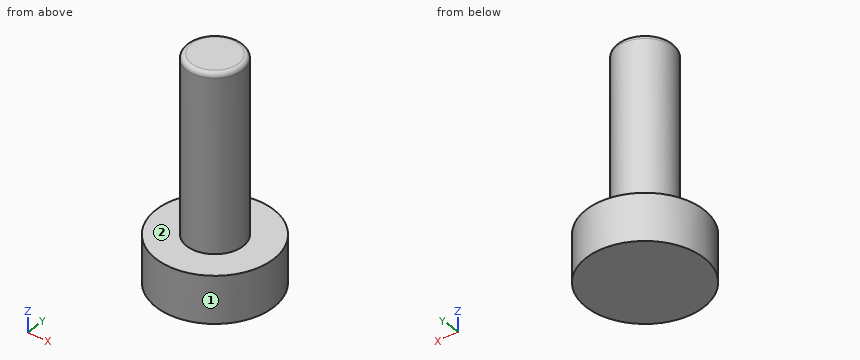
from build123d import *

# Parameters (mm, degrees)
ESQUISSE1_R        = 5
BOSS_EXTRU_1_DEPTH = 4
ESQUISSE2_R        = 2.4
BOSS_EXTRU_2_DEPTH = 15
CONG_1_R           = 0.4


with BuildPart() as part:
    # Esquisse1 → Boss.-Extru.1 (new body)
    with BuildSketch(Plane.XY):
        Circle(ESQUISSE1_R)
    extrude(amount=BOSS_EXTRU_1_DEPTH)

    # Esquisse2 → Boss.-Extru.2 (add)
    with BuildSketch(Plane.XY.offset(4)):
        Circle(ESQUISSE2_R)
    extrude(amount=BOSS_EXTRU_2_DEPTH)

    # Congé1
    cong_1_edges = [part.edges().sort_by_distance(p)[0] for p in [
        (-2.4, 0, 19),
    ]]
    fillet(cong_1_edges, radius=CONG_1_R)


solid = part.part
CAD build for the part. Positions are in the model's coordinates, mm. Face numbers are marked on the shaded views. A direction names the side the tool comes from. Round coordinates to 2 decimals unless told otherwise and drop trailing zeros. Write each loop counter-clockwise with the first axis right and the second up, starting at its lowest first coordinate (ties: lowest second). Pieces come first, ordered by that corner, then holes. Notation, with made-up numbers: M 68.25,14 L 116.25,14 A15 cw 116.25,31 Z; hole C 36.25,-19 d3. An arc over 180 degrees is marked long. Use a Markdown table: item, result. Add a question column.
1. Drill centre lines: probe 1 along Z at (x, y) = (3.5, -1); probe 2 along X at (y, z) = (-1, 18.25). Where is each one in solid material? Low to high.
2. Slice it at D-D on y = -3. Give the cut face in (x, z), then the cut area to 3 significant figures.
3. Slice it at C-C on z = 11.75. Give the cut face in (x, y).
4. Flat gauge pins, fed straight in: P1, Ø4, axis at y = -4, z = 3.5, coming from the -X side; P2, Ø5, axis at x = -2.5, z = 2, coming from the +Y side; P3, Ø2, axis at x = 1, z = 13, coming from the -Y side; P4, Ø6, axis at x = -1, z = 13, coming from the +Y side. Where does each tip first touch, or does it go through?
5. 3-axis set-ups, long thin cutter, end or side, ignore diameter. For the marked faces 1 and 2: which of +Z, -Z, +X, -X, +Y, -Y reach the whole face in a straight line?
6. Slice it at A-A on x = 0. Give the cut face in (y, z).
Reply:
| question | item | result |
|---|---|---|
| 1 | probe 1 | z = 0 to 4 |
| 1 | probe 2 | x = -2.18 to 2.18 |
| 2 | outline | M -4,0 L 4,0 L 4,4 L -4,4 Z |
| 2 | area | 32.0 mm^2 |
| 3 | outline | C 0,0 d4.8 |
| 4 | P1 | stops at x = -4.58 |
| 4 | P2 | stops at y = 5 |
| 4 | P3 | stops at y = -2.4 |
| 4 | P4 | stops at y = 2.4 |
| 5 | face 1 | +Z, -Z |
| 5 | face 2 | +Z |
| 6 | outline | M -5,0 L 5,0 L 5,4 L 2.4,4 L 2.4,18.6 A0.4 ccw 2,19 L -2,19 A0.4 ccw -2.4,18.6 L -2.4,4 L -5,4 Z |
